Can you work these out from the model? Positions are in its coordinate system, mm. A direction names the side the tool comes from. Give positions to 0.01 mm unless a question says otherwise; leave off trailing zeros. Order: outer loops, then holes, each group sorted by start corner. A loop starts at its lowest first (then second) coordinate and runs counter-clockwise, first axis right, second up. Notation, with made-up numbers: (-22, -20) - (11, -20) arc R22 ccw to (11, -7) - close; hole circle Ø10 at (-2, 60). An arc over 180 degrees is marked (long way). Return JSON: item names as keys, results as strings.
```python
from build123d import *

# Parameters (mm, degrees)
F0_R      = 15
F1_DEPTH  = 18.5
F2_T      = -2.5
F3_R      = 12.5
F4_DEPTH  = 12.5
F6_DEPTH  = 10
F8_W      = 6.8951621652
F8_H      = 10.3427423164
F9_DEPTH  = 3
F10_W     = 6.8951621652
F10_H     = 10.3427423164
F11_DEPTH = 18
F12_R     = 3


with BuildPart() as f1:
    # F0 (on Front) → F1 (new body)
    with BuildSketch(Plane.XZ):
        Circle(F0_R)
    extrude(amount=F1_DEPTH)

    # F2
    f2_openings = [f1.faces().sort_by_distance(p)[0] for p in [
        (0, -18.5, 0),
    ]]
    offset(amount=F2_T, openings=f2_openings)

    # F3 (on face) → F4 (join)
    with BuildSketch(Plane.XZ.offset(2.5)):
        Circle(F3_R)
    extrude(amount=F4_DEPTH)

    # F5 (on face) → F6 (cut)
    with BuildSketch(Plane.XZ.offset(15)):
        Polygon((4.7811761408, 3.2363077795), (-0.4121366812, 5.7587738877), (-5.193312822, 2.5224661081), (-4.7811761408, -3.2363077795), (0.4121366812, -5.7587738877), (5.193312822, -2.5224661081), align=None)
    extrude(amount=-F6_DEPTH, mode=Mode.SUBTRACT)

    # F8 (on offset) → F9 (cut)
    with BuildSketch(Plane.YZ.offset(15)):
        with Locations((-9.4354841858, -0.2721771598)):
            Rectangle(F8_W, F8_H)
    extrude(amount=-F9_DEPTH, mode=Mode.SUBTRACT)

    # F10 (on face) → F11 (join)
    with BuildSketch(Plane.YZ.offset(12)):
        with Locations((-9.4354841858, -0.2721771598)):
            Rectangle(F10_W, F10_H)
    extrude(amount=F11_DEPTH)

    # F12
    f12_edges = [f1.edges().sort_by_distance(p)[0] for p in [
        (30, -9.435484, 4.899194),
        (30, -9.435484, -5.443548),
        (30, -5.987903, -0.272177),
        (30, -12.883065, -0.272177),
        (22.088686, -12.883065, 4.899194),
        (21.988701, -12.883065, -5.443548),
        (22.088686, -5.987903, 4.899194),
        (21.988701, -5.987903, -5.443548),
        (-15, 0, 0),
    ]]
    fillet(f12_edges, radius=F12_R)

    # F13: F1 across plane


with BuildPart() as f1_1:
    add(f1.part)
    add(f1.part.mirror(Plane.YZ))


solid = f1_1.part
```
1. Suppose I cut it at C-C (y = -2.25). List the corners of the cut face in (x, z) for me.
Checks:
{"outline": "circle Ø29.81 at (0, 0)"}
2. Thinking about a two-plate mould opening in Z: for faces 5 (the face through (11.923, -16.726, 3.755)), 6 (the face through (-29.145, -6.89, -0.242)), 7 (the face through (-20.678, -12.028, 3.997)), 8 (the face through (0, -5, 0)), which applies, +Z half, -Z half, draft (parallel to the pull), parting line (faces both ways), or undercut?
Checks:
{"face 5": "undercut", "face 6": "draft", "face 7": "+Z half", "face 8": "undercut"}
3. Suppose I cut it at A-A (y = -13.5). List the corners of the cut face in (x, z) for me.
Checks:
{"outline": "circle Ø30 at (0, 0); hole (-5.01, 0) - (-4.81, -2.78) - (-2.51, -4.34) - (0, -5.56) - (2.51, -4.34) - (4.81, -2.78) - (5.01, 0) - (4.81, 2.78) - (2.51, 4.34) - (0, 5.56) - (-2.51, 4.34) - (-4.81, 2.78) - close"}
4. For pin 1 Ø12.5 at (x, z) = (-1, 3) entering from -Y; pin 2 Ø2 at (x, z) = (20.5, -1) entering from +Y; pin 3 Ø6 at (x, y) = (-9.5, -4.5) entering from +Z; pin 4 Ø5 at (x, y) = (-0.5, -3.5) entering from -Z, each with a flat end and sliding along its axis, tell me the tip position at first contact or that it passes through.
Checks:
{"pin 1": "y = -15", "pin 2": "y = -5.99", "pin 3": "z = 13.52", "pin 4": "z = -15"}
5. If I drill on L1, parallel to Z at x = 0, y = -17.8; L2, parallel to Z at x = -23, y = -9, over which ranges is the centre line in solid material (lowest first)? Write a range as [from, to].
Checks:
{"L1": "[-15, -12.5], [12.5, 15]", "L2": "[-5.44, 4.9]"}
6. On a 3-axis mill with a long thin cutter (end or side, diameter ignored), from which of +Z, -Z, +X, -X, +Y, -Y can I reach the whole of each face in a straight line? I mean faces 1 (the face through (20.678, -6.89, 4.044)), 2 (the face through (20.678, -12.028, 3.997)), 3 (the face through (1.27, -10.07, 4.94)), 4 (the face through (-20.6, -6.9, -4.6)). Say none if no direction works.
Checks:
{"face 1": "+Z, +X, +Y", "face 2": "+Z, +X, -Y", "face 3": "-Y", "face 4": "-Z, -X, +Y"}
7. Suppose I cut it at B-B (x = 22). List the corners of the cut face in (y, z) for me, plus the area to 3 significant figures.
Checks:
{"outline": "(-12.88, -2.44) arc R3 ccw to (-9.88, -5.44) - (-8.99, -5.44) arc R3 ccw to (-5.99, -2.44) - (-5.99, 1.9) arc R3 ccw to (-8.99, 4.9) - (-9.88, 4.9) arc R3 ccw to (-12.88, 1.9) - close", "area": "63.6 mm^2"}
